```python
from build123d import *

# Parameters (mm, degrees)
SKETCH1_R                     = 41.5
MAIN_PLATE_DEPTH              = 20
SKETCH3_R                     = 2.5
MOMO_SPARKO_DEPTH             = 63.004032127
SKETCH6_R                     = 4.75
MOMO_SPARKO_SCREW_HEADS_DEPTH = 16
SKETCH7_W                     = 26
SKETCH7_H                     = 26
CUT_EXTRUDE1_DEPTH            = 15
SKETCH8_R                     = 2.5
CUT_EXTRUDE2_DEPTH            = 63.004032127


with BuildPart() as part:
    # Sketch1 → Main Plate (new body)
    with BuildSketch(Plane(origin=(0, 0, 0), x_dir=(1, 0, 0), z_dir=(0, 1, 0))):
        with Locations(Location((0, 0, 0), (0, 0, 270))):
            Circle(SKETCH1_R)
    extrude(amount=MAIN_PLATE_DEPTH)

    # Sketch3 → Momo - Sparko (cut, through all)
    with BuildSketch(Plane(origin=(0, 20, 0), x_dir=(1, 0, 0), z_dir=(0, 1, 0))):
        with Locations(Location((0, 35, 0), (0, 0, 270))):
            Circle(SKETCH3_R)
        with Locations(Location((30.310889132, 17.5, 0), (0, 0, 270))):
            Circle(SKETCH3_R)
        with Locations(Location((30.310889132, -17.5, 0), (0, 0, 270))):
            Circle(SKETCH3_R)
        with Locations(Location((0, -35, 0), (0, 0, 270))):
            Circle(SKETCH3_R)
        with Locations(Location((-30.310889132, -17.5, 0), (0, 0, 270))):
            Circle(SKETCH3_R)
        with Locations(Location((-30.310889132, 17.5, 0), (0, 0, 270))):
            Circle(SKETCH3_R)
    extrude(amount=-MOMO_SPARKO_DEPTH, mode=Mode.SUBTRACT)

    # Sketch6 → Momo - Sparko Screw Heads (cut)
    with BuildSketch(Plane.XZ):
        with Locations(Location((0, 35, 0), (0, 0, 270))):
            Circle(SKETCH6_R)
        with Locations(Location((30.310889132, 17.5, 0), (0, 0, 270))):
            Circle(SKETCH6_R)
        with Locations(Location((30.310889132, -17.5, 0), (0, 0, 270))):
            Circle(SKETCH6_R)
        with Locations(Location((0, -35, 0), (0, 0, 270))):
            Circle(SKETCH6_R)
        with Locations(Location((-30.310889132, -17.5, 0), (0, 0, 270))):
            Circle(SKETCH6_R)
        with Locations(Location((-30.310889132, 17.5, 0), (0, 0, 270))):
            Circle(SKETCH6_R)
    extrude(amount=-MOMO_SPARKO_SCREW_HEADS_DEPTH, mode=Mode.SUBTRACT)

    # Sketch7 → Cut-Extrude1 (cut)
    with BuildSketch(Plane.XZ):
        Rectangle(SKETCH7_W, SKETCH7_H)
    extrude(amount=-CUT_EXTRUDE1_DEPTH, mode=Mode.SUBTRACT)

    # Sketch8 → Cut-Extrude2 (cut, through all)
    with BuildSketch(Plane(origin=(0, 20, 0), x_dir=(1, 0, 0), z_dir=(0, 1, 0))):
        with Locations(Location((0, 0, 0), (0, 0, 270))):
            Circle(SKETCH8_R)
    extrude(amount=-CUT_EXTRUDE2_DEPTH, mode=Mode.SUBTRACT)


solid = part.part
```
Check sheet for the modelled part. Datum: model origin and axes. Units: mm. A direction names the side the tool comes from. Round coordinates to 2 decimals unless told otherwise and drop trailing zeros. Order: outer loops, then holes, each group sorted by start corner. A loop starts at its lowest first (then second) coordinate and runs counter-clockwise, first axis right, second up. Notation, with made-up numbers: M -1,-6 L 42,-6 A19 cw 42,9 Z; hole C -25,41 d4. An arc over 180 degrees is marked long. Answer in a Markdown table with one row per item.
(1) Section check C-C on z = 17.5. Record the boundary of the cut face in (x, y).
Findings:
| item | result |
|---|---|
| outline | M -37.63,0 L -35.06,0 L -35.06,16 L -32.81,16 L -32.81,20 L -37.63,20 Z; M -27.81,16 L -25.56,16 L -25.56,0 L 25.56,0 L 25.56,16 L 27.81,16 L 27.81,20 L -27.81,20 Z; M 32.81,16 L 35.06,16 L 35.06,0 L 37.63,0 L 37.63,20 L 32.81,20 Z |
(2) Gauge pin test, flat ends, axial feed: pin 1 (1 mm diameter, centred on x = 26.5, y = 8.5, fed in from -Z); pin 2 (2 mm diameter, centred on y = 10.5, z = 19, fed in from -X); pin 3 (4 mm diameter, centred on x = 10, y = 5, fed in from +Z); pin 4 (11 mm diameter, centred on x = 30.31, z = 17.5, fed in from +Y). Record the tip position at first contact, or that the pin passes through.
Findings:
| item | result |
|---|---|
| pin 1 | stops at z = -32.35 |
| pin 2 | stops at x = -37.39 |
| pin 3 | stops at z = 40.72 |
| pin 4 | stops at y = 20 |
(3) Draft check along Z on faces 3 (the flat face through (-9, 20, -1)), 4 (the cylindrical face through (12.465, 9.86, 39.584)), 5 (the cylindrical face through (-34.948, 7.888, 18.53)). Enter one of: +Z half, -Z half, draft (parallel to the pull), parting line (faces both ways), or undercut.
Findings:
| item | result |
|---|---|
| face 3 | draft |
| face 4 | parting line |
| face 5 | undercut |
(4) Set-up check for faces 1 (the cylindrical face through (-0.96, 18.03, 37.31)), 2 (the flat face through (0, 7, 13)): record each of +Z, -Z, +X, -X, +Y, -Y from which the full face is reachable in a straight line by a thin tool's end or side.
Findings:
| item | result |
|---|---|
| face 1 | +Y, -Y |
| face 2 | -Y |
(5) Section check A-A on x = 0. Record the boundary of the cut face in (y, z).
Findings:
| item | result |
|---|---|
| outline | M 0,-41.5 L 20,-41.5 L 20,-37.5 L 16,-37.5 L 16,-39.75 L 0,-39.75 Z; M 0,-30.25 L 16,-30.25 L 16,-32.5 L 20,-32.5 L 20,-2.5 L 15,-2.5 L 15,-13 L 0,-13 Z; M 0,13 L 15,13 L 15,2.5 L 20,2.5 L 20,32.5 L 16,32.5 L 16,30.25 L 0,30.25 Z; M 0,39.75 L 16,39.75 L 16,37.5 L 20,37.5 L 20,41.5 L 0,41.5 Z |
(6) Material ranges on line 1 along X through (y, z) = (7.5, 14.5); line 2 along X through (y, z) = (15.25, -17); line 3 along X through (y, z) = (18.4, 35), recorded low to high. Write a range as from..to.
Findings:
| item | result |
|---|---|
| line 1 | x = -38.88..-33.99, -26.63..26.63, 33.99..38.88 |
| line 2 | x = -37.86..-35.03, -25.59..25.59, 35.03..37.86 |
| line 3 | x = -22.3..-2.5, 2.5..22.3 |
(7) Section check B-B on z = -35.5. Record the boundary of the cut face in (x, y).
Findings:
| item | result |
|---|---|
| outline | M -21.49,0 L -4.72,0 L -4.72,16 L -2.45,16 L -2.45,20 L -21.49,20 Z; M 2.45,16 L 4.72,16 L 4.72,0 L 21.49,0 L 21.49,20 L 2.45,20 Z |
(8) Section check D-D on y = 8.75. Record the boundary of the cut face in (x, z), plus the area to 3 significant figures.
Findings:
| item | result |
|---|---|
| outline | C 0,0 d83; hole C -30.31,-17.5 d9.5; hole C -30.31,17.5 d9.5; hole M -13,-13 L 13,-13 L 13,13 L -13,13 Z; hole C 0,-35 d9.5; hole C 0,35 d9.5; hole C 30.31,-17.5 d9.5; hole C 30.31,17.5 d9.5 |
| area | 4,310 mm^2 |
